Could you check a few things on this model? Use its own coordinates, in mm. Give positions to 0.01 mm unless a question says otherwise; leave off trailing zeros. Order: outer loops, then holes, each group sorted by start corner. A loop starts at its lowest first (then second) coordinate and runs counter-clockwise, first axis right, second up. Notation, with made-up numbers: (37.5, -25.5) -> (55.5, -25.5) arc R35 cw to (55.5, 6.5) -> close; hole circle Ø3 at (-17, -20.75). An arc over 180 degrees is marked (long way). One line per item, written item: value.
Autodesk Inventor part; units mm, degrees
ref_plane "YZ Plane" through (0, 0, 0) normal (1, 0, 0) x (0, 1, 0)
ref_plane "XZ Plane" through (0, 0, 0) normal (0, 1, 0) x (-1, 0, 0)
ref_plane "XY Plane" through (0, 0, 0) normal (0, 0, 1) x (1, 0, 0)
sketch "Sketch1" plane through (0, 0, 0) normal (0, 0, 1) x (1, 0, 0)
  line L0 (0, 4.445) -> (0, -4.445)
  arc A0 (0, 3.175) -> (0, -3.175) centre (0, 0) ccw
  circle A1 centre (0, 0) radius 1.5875
  line L1 (0, 3.175) -> (0, -3.175)
  dimension "d0" = 3.175
  dimension "d1" = 3.175
revolve "Revolution1" add sketch "Sketch1" angle 360 about axis through (0, 0, 0) along (0, -1, 0) picked at (-0.4775, -0.3807) contours L0 A1 A0 | L0 A1
extrude "Extrusion1" cut sketch "Sketch1" along normal mid plane 6.35 contours A1 L0 | L0 A1
scale "Scale1" factors (10, 10, 10) then translate (0, 0, 0) bodies 1
properties part number "ball"
1) Suppose I cut it at A-A, the plane y = 0. Write out the boundary of the cut face in (x, z) (3 decimals), then the cut area to 3 significant figures.
Answer below:
outline: (-15.875, -27.496) -> (-15.875, 27.496) arc R31.75 ccw to start; (15.875, -27.496) arc R31.75 ccw to (15.875, 27.496) -> close
area: 1,240 mm2
2) For P1, Ø5, axis at x = -3, z = -14, coming from the +Y side; P2, Ø4, axis at x = 22, y = -2, coming from the +Z side; P3, Ø1, axis at x = 17.5, y = -8, coming from the -Z side; P4, Ø10, axis at x = 5.5, y = 3.5, coming from the -Z side (1 decimal), each with a flat end and sliding along its axis, tell me the tip position at first contact or that it passes through.
Answer below:
P1: stops at y = 29.47
P2: stops at z = 24.59
P3: stops at z = -25.63
P4: passes through
3) Suppose I cut it at D-D, the plane x = -25. Write out the boundary of the cut face in (y, z), then the cut area to 3 significant figures.
Answer below:
outline: circle Ø39.14 at (0, 0)
area: 1,200 mm2
4) Suppose I cut it at C-C, the plane z = -11. Write out the boundary of the cut face in (x, y) (3 decimals), then the cut area to 3 significant figures.
Answer below:
outline: circle Ø59.567 at (0, 0); hole circle Ø31.75 at (0, 0)
area: 2,000 mm2
